Autodesk Inventor part; units mm, degrees
ref_plane "YZ Plane" through (0, 0, 0) normal (1, 0, 0) x (0, 1, 0)
ref_plane "XZ Plane" through (0, 0, 0) normal (0, 1, 0) x (-1, 0, 0)
ref_plane "XY Plane" through (0, 0, 0) normal (0, 0, 1) x (1, 0, 0)
sketch "Sketch1" plane through (0, 0, 0) normal (0, 0, 1) x (1, 0, 0)
  circle A0 centre (0, 0) radius 28.575
  circle A1 centre (0, 0) radius 6.35
  line L0 (-1.5875, 4.7625) -> (1.5875, 4.7625)
  line L1 (1.5875, 4.7625) -> (1.5875, 7.9375)
  line L2 (1.5875, 7.9375) -> (-1.5875, 7.9375)
  line L3 (-1.5875, 7.9375) -> (-1.5875, 4.7625)
  line L4 (1.5875, 6.35) -> (-1.5875, 6.35)
  circle A2 centre (0, 0) radius 12.7
  point P0 (0, 4.7625)
  point P1 (0, 23.8125)
  point P2 (-20.6222, 11.9063)
  point P3 (-20.6222, -11.9062)
  point P4 (0, -23.8125)
  point P5 (20.6222, -11.9063)
  point P6 (20.6222, 11.9062)
  dimension "d0" = 57.15
  dimension "d1" = 12.7
  dimension "d2" = 3.175
  dimension "d3" = 3.175
  dimension "d6" = 360
  dimension "d8" = 23.8125
  dimension "d9" = 25.4
extrude "Extrusion1" add sketch "Sketch1" against normal blind 6.35 contours A0 | A2
extrude "Extrusion2" add sketch "Sketch1" along normal blind 19.05 contours A2
hole "Hole1" at (0, 23.8125, 0) at (-20.6222, 11.9063, 0) at (-20.6222, -11.9062, 0) at (0, -23.8125, 0) at (20.6222, -11.9063, 0) at (20.6222, 11.9062, 0) direction (0, 0, -1) diameter 5.1816 depth 25.4 tip angle 118
properties part number "wheel hub"
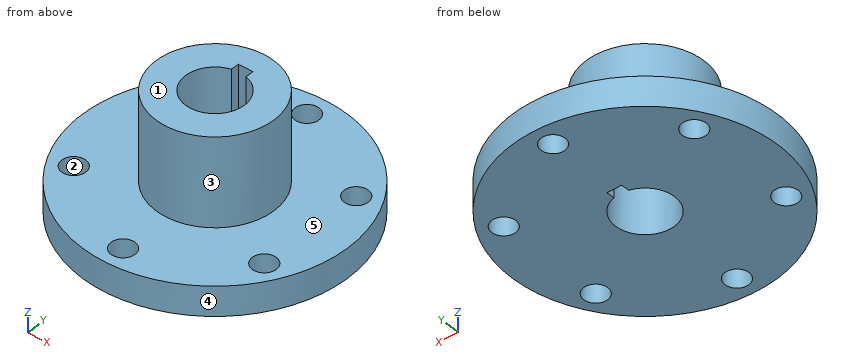
Verification items for the finished model (mm, model axes). Face numbers are marked on the shaded views. A direction names the side the tool comes from. Give positions to 0.01 mm unless a question says otherwise; leave off trailing zeros. Write each loop counter-clockwise with the first axis right and the second up, starting at its lowest first coordinate (ties: lowest second). Pieces come first, ordered by that corner, then holes. Notation, with made-up numbers: M -35.75,73 L -15.75,73 A21 ccw -15.75,78 Z; hole C 8,61.25 d4. An arc over 180 degrees is marked long. Write item = value, one per line.
(1) Sectioned sample at D-D (y = 10). Record the cut outline in (x, z), then the cut area to 3 significant figures.
Found:
outline = M -26.77,-6.35 L -22.38,-6.35 L -22.38,0 L -26.77,0 Z; M -18.87,-6.35 L 18.87,-6.35 L 18.87,0 L 7.83,0 L 7.83,19.05 L -7.83,19.05 L -7.83,0 L -18.87,0 Z; M 22.38,-6.35 L 26.77,-6.35 L 26.77,0 L 22.38,0 Z
area = 594 mm2
(2) Sectioned sample at B-B (x = 0). Give the number of separate pieces and of enclosed holes in the cut face, then the cut area to 3 significant figures.
Found:
separate_pieces = 4
enclosed_holes = 0
area = 418 mm2
(3) Sectioned sample at A-A (y = 0). Record the cut outline in (x, z) (3 decimals), then the cut area to 3 significant figures.
Found:
outline = M -28.575,-6.35 L -6.35,-6.35 L -6.35,19.05 L -12.7,19.05 L -12.7,0 L -28.575,0 Z; M 6.35,-6.35 L 28.575,-6.35 L 28.575,0 L 12.7,0 L 12.7,19.05 L 6.35,19.05 Z
area = 524 mm2
(4) Material ranges on line 1 (Y direction, x = 0, z = 11); line 2 (Z direction, x = 22, y = 7.5); line 3 (X direction, y = 4.5, z = 15), recorded low to high.
Found:
line_1 = -12.7 to -6.35, 7.94 to 12.7
line_2 = -6.35 to 0
line_3 = -11.88 to -4.48, 4.48 to 11.88
(5) Sectioned sample at C-C (z = 11.75). Record the cut outline in (x, y).
Found:
outline = C 0,0 d25.4; hole M -1.59,6.15 A6.35 ccw long 1.59,6.15 L 1.59,7.94 L -1.59,7.94 Z
(6) Go/stop test with flat-tipped pins: pin 1 Ø4 at (x, z) = (1.5, 15) entering from +Y; pin 2 Ø8.5 at (x, y) = (20.62, 11.91) entering from +Z; pin 3 Ø6 at (x, y) = (20.62, -11.91) entering from -Z; pin 4 Ø2 at (y, z) = (-10, -1.5) entering from +X. Record where each tip stops, or that it passes through.
Found:
pin_1 = 12.7
pin_2 = 0
pin_3 = -6.35
pin_4 = 27.12
(7) Draft check along Y on the marked faces 1, 2 and 3. Enter one of: released by +Y, released by -Y, zero draft, split by the parting line, or undercut.
Found:
face_1 = zero draft
face_2 = undercut
face_3 = split by the parting line
(8) Access from +Z, -Z, +X, -X, +Y, -Y to the whole of each face (thin tool, end or side, straight path). Record for the marked faces 4 and 5.
Found:
face_4 = +Z, -Z
face_5 = +Z
